from build123d import *

# Parameters (mm, degrees)
SKETCH1_W           = 90
SKETCH1_H           = 60
BOSS_EXTRUDE1_DEPTH = 5
SKETCH3_R           = 9.25
CUT_EXTRUDE2_DEPTH  = 5
SKETCH4_W           = 17.5
SKETCH4_H           = 17.5
CUT_EXTRUDE3_DEPTH  = 5
SKETCH5_R           = 1.75
CUT_EXTRUDE4_DEPTH  = 5
SKETCH6_R           = 5
SKETCH6_R_2         = 1
CUT_EXTRUDE5_DEPTH  = 10
FILLET1_R           = 10
SKETCH7_W           = 5
SKETCH7_H           = 11
SKETCH7_H_2         = 12
SKETCH7_R           = 1.5
CUT_EXTRUDE6_DEPTH  = 5


with BuildPart() as part:
    # Sketch1 → Boss-Extrude1 (new body)
    with BuildSketch(Plane.XY):
        Rectangle(SKETCH1_W, SKETCH1_H)
    extrude(amount=BOSS_EXTRUDE1_DEPTH)

    # Sketch3 → Cut-Extrude2 (cut)
    with BuildSketch(Plane.XY.offset(5)):
        with Locations((0, 15)):
            Circle(SKETCH3_R)
    extrude(amount=-CUT_EXTRUDE2_DEPTH, mode=Mode.SUBTRACT)

    # Sketch4 → Cut-Extrude3 (cut)
    with BuildSketch(Plane.XY.offset(5)):
        with Locations((0, 15)):
            Rectangle(SKETCH4_W, SKETCH4_H)
    extrude(amount=-CUT_EXTRUDE3_DEPTH, mode=Mode.SUBTRACT)

    # Sketch5 → Cut-Extrude4 (cut)
    with BuildSketch(Plane.XY.offset(5)):
        with Locations((-8.75, 15)):
            Circle(SKETCH5_R)
        with Locations((8.75, 15)):
            Circle(SKETCH5_R)
    extrude(amount=-CUT_EXTRUDE4_DEPTH, mode=Mode.SUBTRACT)

    # Sketch6 → Cut-Extrude5 (cut)
    with BuildSketch(Plane.XY.offset(5)):
        with Locations((-22.5, 3)):
            Circle(SKETCH6_R)
        with Locations((22.5, 3)):
            Circle(SKETCH6_R)
        with Locations((-20, -12.5)):
            Circle(SKETCH6_R_2)
        with Locations((0, -12.5)):
            Circle(SKETCH6_R_2)
        with Locations((20, -12.5)):
            Circle(SKETCH6_R_2)
    extrude(amount=-CUT_EXTRUDE5_DEPTH, mode=Mode.SUBTRACT)

    # Fillet1
    # the kernel refuses this fillet: 10 mm, written as the material it takes off along each edge
    with BuildSketch(Plane(origin=(9.089285714, 13.283204962, -3.318254218), x_dir=(0.8690606948283255, 0.4947054767278286, 0), z_dir=(0, 0, 1))) as fillet1_piece_1:
        with BuildLine():
            CenterArc((4.277170512, -9.484831943), FILLET1_R, 108.471170307, 12.906966453)
            Line((-0.929668401, -0.947336494), (-1.033805179, -0.776586585))
            ThreePointArc((-1.033805179, -0.776586585), (-0.590566588, -0.350280804), (-0.152428823, 0.129481481))
            Line((-0.152428823, 0.129481481), (0.063365489, 0.189696639))
            ThreePointArc((0.063365489, 0.189696639), (0.554448029, 0.10984559), (1.04553057, 0.189696639))
            Line((1.04553057, 0.189696639), (1.108896059, 0))
        make_face()
    extrude(amount=11.636508437, mode=Mode.SUBTRACT)
    with BuildSketch(Plane(origin=(9.089285714, 16.716795038, -3.318254218), x_dir=(-0.255620645644957, 0.9667771643559105, 0), z_dir=(0, 0, 1))) as fillet1_piece_2:
        with BuildLine():
            CenterArc((3.77380457, -9.696113842), FILLET1_R, 104.1611678, 12.906966453)
            Line((-0.776692771, -0.791453605), (-0.867702718, -0.6133604))
            ThreePointArc((-0.867702718, -0.6133604), (-0.466746599, -0.318788775), (-0.179774835, 0.087641364))
            Line((-0.179774835, 0.087641364), (0.014349207, 0.199484586))
            ThreePointArc((0.014349207, 0.199484586), (0.663650844, 0.176162125), (1.27837163, 0.193922277))
            Line((1.27837163, 0.193922277), (1.327301687, 0))
        make_face()
    extrude(amount=11.636508437, mode=Mode.SUBTRACT)
    with BuildSketch(Plane(origin=(-9.089285714, 16.716795038, -3.318254218), x_dir=(0.25562064564495884, 0.9667771643559101, 0), z_dir=(0, 0, 1))) as fillet1_piece_3:
        with BuildLine():
            CenterArc((3.77380457, 9.696113842), FILLET1_R, 242.931865747, 12.906966453)
            Line((-0.776692771, 0.791453605), (-0.867702718, 0.6133604))
            ThreePointArc((-0.867702718, 0.6133604), (-0.466746599, 0.318788775), (-0.179774835, -0.087641364))
            Line((-0.179774835, -0.087641364), (0.014349207, -0.199484586))
            ThreePointArc((0.014349207, -0.199484586), (0.663650844, -0.176162125), (1.27837163, -0.193922277))
            Line((1.27837163, -0.193922277), (1.327301687, 0))
        make_face()
    extrude(amount=11.636508437, mode=Mode.SUBTRACT)
    with BuildSketch(Plane(origin=(-9.089285714, 13.283204962, -3.318254218), x_dir=(-0.8690606948283244, 0.4947054767278305, 0), z_dir=(0, 0, 1))) as fillet1_piece_4:
        with BuildLine():
            CenterArc((4.277170512, 9.484831943), FILLET1_R, 238.62186324, 12.906966453)
            Line((-0.929668401, 0.947336494), (-1.033805179, 0.776586585))
            ThreePointArc((-1.033805179, 0.776586585), (-0.590566588, 0.350280804), (-0.152428823, -0.129481481))
            Line((-0.152428823, -0.129481481), (0.063365489, -0.189696639))
            ThreePointArc((0.063365489, -0.189696639), (0.554448029, -0.10984559), (1.04553057, -0.189696639))
            Line((1.04553057, -0.189696639), (1.108896059, 0))
        make_face()
    extrude(amount=11.636508437, mode=Mode.SUBTRACT)

    # Sketch7 → Cut-Extrude6 (cut)
    with BuildSketch(Plane.XY.offset(5)):
        with Locations((-37.5, 29.5)):
            Rectangle(SKETCH7_W, SKETCH7_H)
        with Locations((-37.5, 5)):
            Rectangle(SKETCH7_W, SKETCH7_H_2)
        with Locations((-37.5, -19.5)):
            Rectangle(SKETCH7_W, SKETCH7_H)
        with Locations((-37.5, 17.5)):
            Circle(SKETCH7_R)
        with Locations((-37.5, -7.5)):
            Circle(SKETCH7_R)
    cut_extrude6 = extrude(amount=-CUT_EXTRUDE6_DEPTH, mode=Mode.SUBTRACT)

    # Mirror1: Cut-Extrude6 across plane
    add(cut_extrude6.mirror(Plane(origin=(0, 0, 0), x_dir=(0, 0, 1), z_dir=(1, 0, 0))), mode=Mode.SUBTRACT)


solid = part.part
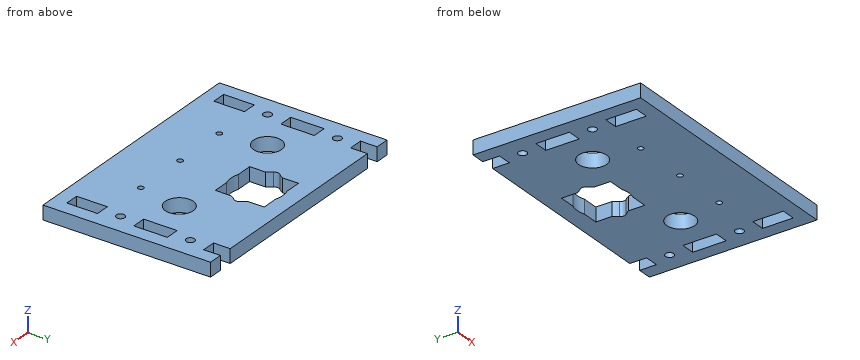
Can you work these out from the model? Positions are in its coordinate system, mm. Round coordinates to 2 decimals unless told otherwise and drop trailing zeros. Order: outer loops, then holes, each group sorted by start corner. A loop starts at its lowest first (then second) coordinate and runs counter-clockwise, first axis right, second up. Notation, with made-up numbers: (-31.75, 49.5) - (9.25, 49.5) arc R20 cw to (9.25, 83.5) - close; hole circle Ø2 at (8.25, 62). An arc over 180 degrees is marked (long way). Answer in a Markdown table with one row per item.
(1) Suppose I cut it at C-C, the plane y = 15. Please give me the cut outline in (x, z).
From the geometry:
| item | result |
|---|---|
| outline | (-45, 0) - (-10.5, 0) - (-10.5, 5) - (-45, 5) - close; (10.5, 0) - (45, 0) - (45, 5) - (10.5, 5) - close |
(2) Suppose I cut it at A-A, the plane y = -12.5. Please give me the cut outline in (x, z), plus the area to 3 significant figures.
From the geometry:
| item | result |
|---|---|
| outline | (-45, 0) - (-21, 0) - (-21, 5) - (-45, 5) - close; (-19, 0) - (-1, 0) - (-1, 5) - (-19, 5) - close; (1, 0) - (19, 0) - (19, 5) - (1, 5) - close; (21, 0) - (45, 0) - (45, 5) - (21, 5) - close |
| area | 420 mm2 |
(3) Please list where these lines run through material, in increasing order: L1, parallel to X at y = 25.5, z = 1.25; L2, parallel to Y at x = -37.5, z = 2.9; L3, parallel to Y at x = 20, z = 1.65. Write a range as from..to.
From the geometry:
| item | result |
|---|---|
| L1 | x = -45..-40, -35..35, 40..45 |
| L2 | y = -30..-25, -14..-9, -6..-1, 11..16, 19..24 |
| L3 | y = -30..-13.5, -11.5..-1.33, 7.33..30 |
(4) Suppose I cut it at B-B, the plane x = -37.5. Please give me the cut outline in (y, z), plus the area to 3 significant figures.
From the geometry:
| item | result |
|---|---|
| outline | (-30, 0) - (-25, 0) - (-25, 5) - (-30, 5) - close; (-14, 0) - (-9, 0) - (-9, 5) - (-14, 5) - close; (-6, 0) - (-1, 0) - (-1, 5) - (-6, 5) - close; (11, 0) - (16, 0) - (16, 5) - (11, 5) - close; (19, 0) - (24, 0) - (24, 5) - (19, 5) - close |
| area | 125 mm2 |
(5) For P1, Ø2, axis at x = -35.5, z = 2, coming from the +Y side; P2, Ø1.2, axis at x = 0, y = -12.5, coming from the -Z side; P3, Ø1.5, axis at x = -36.5, z = 2.5, coming from the +Y side, each with a flat end and sliding along its axis, tell me the tip position at first contact or that it passes through.
From the geometry:
| item | result |
|---|---|
| P1 | stops at y = 30 |
| P2 | passes through |
| P3 | stops at y = 24 |
(6) Suppose I cut it at D-D, the plane x = -22.5. Please give me the cut outline in (y, z), plus the area to 3 significant figures.
From the geometry:
| item | result |
|---|---|
| outline | (-30, 0) - (-2, 0) - (-2, 5) - (-30, 5) - close; (8, 0) - (30, 0) - (30, 5) - (8, 5) - close |
| area | 250 mm2 |
